Autodesk Inventor part; units mm, degrees
ref_plane "YZ Plane" through (0, 0, 0) normal (1, 0, 0) x (0, 1, 0)
ref_plane "XZ Plane" through (0, 0, 0) normal (0, 1, 0) x (-1, 0, 0)
ref_plane "XY Plane" through (0, 0, 0) normal (0, 0, 1) x (1, 0, 0)
sketch "Sketch1" plane through (0, 0, 0) normal (0, 1, 0) x (-1, 0, 0)
  line L0 (-45, 90) -> (45, 90)
  line L1 (45, 90) -> (45, -90)
  line L2 (45, -90) -> (-45, -90)
  line L3 (-45, -90) -> (-45, 90)
  line L4 (-45, 90) -> (45, -90) construction
  line L5 (45, 90) -> (-45, -90) construction
  point P0 (0, 0)
  dimension "d0" = 180
  dimension "d1" = 90
extrude "Extrusion1" add sketch "Sketch1" along normal blind 20
sketch "Sketch2" plane through (-45, 0, 90) normal (0, 0, 1) x (1, 0, 0)
  circle A0 centre (65, 10) radius 7.5
  circle A1 centre (25, 10) radius 7.5
  point P0 (45, 0)
  dimension "d4" = 20
  dimension "d5" = 20
  dimension "d6" = 10
  dimension "d7" = 10
  dimension "d8" = 15
  dimension "d9" = 15
extrude "Extrusion2" cut sketch "Sketch2" against normal through all
properties part number "Motor Platform"
Can you work these out from the model? Positions are in its coordinate system, mm. Round coordinates to 2 decimals unless told otherwise and drop trailing zeros. Loops run counter-clockwise (first coordinate to the right, second up) from the corner with the lowest first, then second, coordinate; pieces in that order, holes last. Notation, with made-up numbers: M 11,-30 L 35,-30 A23 ccw 35,-1 Z; hole C 76.5,53.25 d8. An arc over 180 degrees is marked long. Answer as a JSON object with one key per item and string values. Group by question number.
Q1. Imagine slicing it at B-B, the plane y = 10. Please give me the cut outline in (x, z), then the cut area to 3 significant figures.
Q2. Imagine slicing it at A-A, the plane x = -20. Please give me the cut outline in (y, z), then the cut area to 3 significant figures.
Q3. Please list where these lines run through material, in increasing order: L1, parallel to X at y = 9.75, z = 19; L2, parallel to Y at x = 20, z = -1.5; L3, parallel to X at y = 5.25, z = -0.5.
Q4. Imagine slicing it at C-C, the plane z = -14. Please give me the cut outline in (x, y).
Q5. We'd pull the mould along Y, two halves only. Please class faces 1 (the flat face through (-45, 10, 1)), 2 (the flat face through (1, 0, 1)), 3 (the cylindrical face through (14.048, 5.436, 1.26)): +Y half, -Y half, draft (parallel to the pull), parting line (faces both ways), or undercut.
Findings:
{
 "1": {"outline": "M -45,-90 L -27.5,-90 L -27.5,90 L -45,90 Z; M -12.5,-90 L 12.5,-90 L 12.5,90 L -12.5,90 Z; M 27.5,-90 L 45,-90 L 45,90 L 27.5,90 Z", "area": "10,800 mm2"},
 "2": {"outline": "M 0,-90 L 2.5,-90 L 2.5,90 L 0,90 Z; M 17.5,-90 L 20,-90 L 20,90 L 17.5,90 Z", "area": "900 mm2"},
 "3": {"L1": "x = -45 to -27.5, -12.5 to 12.5, 27.5 to 45", "L2": "y = 0 to 2.5, 17.5 to 20", "L3": "x = -45 to -25.8, -14.2 to 14.2, 25.8 to 45"},
 "4": {"outline": "M -45,0 L 45,0 L 45,20 L -45,20 Z; hole C -20,10 d15; hole C 20,10 d15"},
 "5": {"face 1": "draft", "face 2": "-Y half", "face 3": "undercut"}
}
